from build123d import *

# Parameters (mm, degrees)
SKETCH1_R                 = 3.4
F_40_X_40L_X_R4_5_1_DEPTH = 300


with BuildPart() as part:
    # Sketch1 → 铝型材 40 X 40L X R4.5(1) (new body)
    with BuildSketch(Plane.XY.offset(-151.807228916)):
        with BuildLine():
            Line((-5.1, 20), (-5.1, 19.5))
            Line((-5.1, 19.5), (-4.1, 19.5))
            Line((-4.1, 19.5), (-4.1, 17))
            Line((-4.1, 17), (-6.1, 17))
            Line((-6.1, 17), (-6.1, 18.5))
            Line((-6.1, 18.5), (-10.3, 18.5))
            Line((-10.3, 18.5), (-10.3, 11.3))
            Line((-10.3, 11.3), (-5, 6))
            Line((-5, 6), (5, 6))
            Line((5, 6), (10.3, 11.3))
            Line((10.3, 11.3), (10.3, 18.5))
            Line((10.3, 18.5), (6.1, 18.5))
            Line((6.1, 18.5), (6.1, 17))
            Line((6.1, 17), (4.1, 17))
            Line((4.1, 17), (4.1, 19.5))
            Line((4.1, 19.5), (5.1, 19.5))
            Line((5.1, 19.5), (5.1, 20))
            Line((5.1, 20), (15.5, 20))
            ThreePointArc((15.5, 20), (18.681980515, 18.681980515), (20, 15.5))
            Line((20, 15.5), (20, 5.1))
            Line((20, 5.1), (19.5, 5.1))
            Line((19.5, 5.1), (19.5, 4.1))
            Line((19.5, 4.1), (17, 4.1))
            Line((17, 4.1), (17, 6.1))
            Line((17, 6.1), (18.5, 6.1))
            Line((18.5, 6.1), (18.5, 10.3))
            Line((18.5, 10.3), (11.3, 10.3))
            Line((11.3, 10.3), (6, 5))
            Line((6, 5), (6, -5))
            Line((6, -5), (11.3, -10.3))
            Line((11.3, -10.3), (18.5, -10.3))
            Line((18.5, -10.3), (18.5, -6.1))
            Line((18.5, -6.1), (17, -6.1))
            Line((17, -6.1), (17, -4.1))
            Line((17, -4.1), (19.5, -4.1))
            Line((19.5, -4.1), (19.5, -5.1))
            Line((19.5, -5.1), (20, -5.1))
            Line((20, -5.1), (20, -15.5))
            ThreePointArc((20, -15.5), (18.681980515, -18.681980515), (15.5, -20))
            Line((15.5, -20), (5.1, -20))
            Line((5.1, -20), (5.1, -19.5))
            Line((5.1, -19.5), (4.1, -19.5))
            Line((4.1, -19.5), (4.1, -17))
            Line((4.1, -17), (6.1, -17))
            Line((6.1, -17), (6.1, -18.5))
            Line((6.1, -18.5), (10.3, -18.5))
            Line((10.3, -18.5), (10.3, -11.3))
            Line((10.3, -11.3), (5, -6))
            Line((5, -6), (-5, -6))
            Line((-5, -6), (-10.3, -11.3))
            Line((-10.3, -11.3), (-10.3, -18.5))
            Line((-10.3, -18.5), (-6.1, -18.5))
            Line((-6.1, -18.5), (-6.1, -17))
            Line((-6.1, -17), (-4.1, -17))
            Line((-4.1, -17), (-4.1, -19.5))
            Line((-4.1, -19.5), (-5.1, -19.5))
            Line((-5.1, -19.5), (-5.1, -20))
            Line((-5.1, -20), (-15.5, -20))
            ThreePointArc((-15.5, -20), (-18.681980515, -18.681980515), (-20, -15.5))
            Line((-20, -15.5), (-20, -5.1))
            Line((-20, -5.1), (-19.5, -5.1))
            Line((-19.5, -5.1), (-19.5, -4.1))
            Line((-19.5, -4.1), (-17, -4.1))
            Line((-17, -4.1), (-17, -6.1))
            Line((-17, -6.1), (-18.5, -6.1))
            Line((-18.5, -6.1), (-18.5, -10.3))
            Line((-18.5, -10.3), (-11.3, -10.3))
            Line((-11.3, -10.3), (-6, -5))
            Line((-6, -5), (-6, 5))
            Line((-6, 5), (-11.3, 10.3))
            Line((-11.3, 10.3), (-18.5, 10.3))
            Line((-18.5, 10.3), (-18.5, 6.1))
            Line((-18.5, 6.1), (-17, 6.1))
            Line((-17, 6.1), (-17, 4.1))
            Line((-17, 4.1), (-19.5, 4.1))
            Line((-19.5, 4.1), (-19.5, 5.1))
            Line((-19.5, 5.1), (-20, 5.1))
            Line((-20, 5.1), (-20, 15.5))
            ThreePointArc((-20, 15.5), (-18.681980515, 18.681980515), (-15.5, 20))
            Line((-15.5, 20), (-5.1, 20))
        make_face()
        Circle(SKETCH1_R, mode=Mode.SUBTRACT)
        with BuildLine():
            Line((11.8, 17.5), (15, 17.5))
            ThreePointArc((15, 17.5), (16.767766953, 16.767766953), (17.5, 15))
            Line((17.5, 15), (17.5, 11.8))
            Line((17.5, 11.8), (11.8, 11.8))
            Line((11.8, 11.8), (11.8, 17.5))
        make_face(mode=Mode.SUBTRACT)
        with BuildLine():
            Line((-15, 17.5), (-11.8, 17.5))
            Line((-11.8, 17.5), (-11.8, 11.8))
            Line((-11.8, 11.8), (-17.5, 11.8))
            Line((-17.5, 11.8), (-17.5, 15))
            ThreePointArc((-17.5, 15), (-16.767766953, 16.767766953), (-15, 17.5))
        make_face(mode=Mode.SUBTRACT)
        with BuildLine():
            Line((-17.5, -11.8), (-11.8, -11.8))
            Line((-11.8, -11.8), (-11.8, -17.5))
            Line((-11.8, -17.5), (-15, -17.5))
            ThreePointArc((-15, -17.5), (-16.767766953, -16.767766953), (-17.5, -15))
            Line((-17.5, -15), (-17.5, -11.8))
        make_face(mode=Mode.SUBTRACT)
        with BuildLine():
            Line((11.8, -11.8), (17.5, -11.8))
            Line((17.5, -11.8), (17.5, -15))
            ThreePointArc((17.5, -15), (16.767766953, -16.767766953), (15, -17.5))
            Line((15, -17.5), (11.8, -17.5))
            Line((11.8, -17.5), (11.8, -11.8))
        make_face(mode=Mode.SUBTRACT)
    extrude(amount=F_40_X_40L_X_R4_5_1_DEPTH)


solid = part.part
Build history of the part. All positions in model axes, mm. A direction names the side the tool comes from. Round coordinates to 2 decimals unless told otherwise and drop trailing zeros. Write each loop counter-clockwise with the first axis right and the second up, starting at its lowest first coordinate (ties: lowest second). Pieces come first, ordered by that corner, then holes. Notation, with made-up numbers: M 83.25,45.5 L 113.25,45.5 A15 ccw 113.25,56.5 Z; hole C 21,-14 d5. An arc over 180 degrees is marked long. Answer as a JSON object with one key per item and string values. Group by question number.
(1) Cut at C-C (z = -110). Give the number of separate pieces and of enclosed holes in the cut face, and give its area (3 significant figures).
(2) Cut at A-A (x = 0). Give the cut face in (y, z).
(3) Which spindle directions (+Z, -Z, +X, -X, +Y, -Y) get a long thin tool onto all of the face, cutting with end or side? Do faces 4 (the flat face through (9, 8, -4)), 5 (the flat face through (10, -20, -4)). Say none if no direction does.
(4) Drill centre lines: L1, parallel to Y at x = 4.5, z = -18; L2, parallel to X at y = 14, z = 99; L3, parallel to Y at x = -15.5, z = 5.5. Where is each one in solid material? Low to high.
(5) Mould opens along Y. For faces 1 (the flat face through (-11.8, -15, -4)), 2 (the flat face through (-3, 3, -151.807)), 3 (the flat face through (-10, -20, -4)) say: pulls with the +Y half, pulls with the -Y half, needs draft (parallel to the pull), parting line crosses it, or undercut.
(6) Flat gauge pins, fed straight in: pin 1 (1 mm diameter, centred on y = -0.5, z = -24.5, fed in from -X); pin 2 (0.5 mm diameter, centred on y = -4.5, z = 9.5, fed in from +X). Where does each tip first touch, or does it go through?
Responses:
{
 "1": {"separate pieces": "1", "enclosed holes": "5", "area": "475 mm2"},
 "2": {"outline": "M -6,-151.81 L -3.4,-151.81 L -3.4,148.19 L -6,148.19 Z; M 3.4,-151.81 L 6,-151.81 L 6,148.19 L 3.4,148.19 Z"},
 "3": {"face 4": "+Z, -Z", "face 5": "+Z, -Z, +X, -X, -Y"},
 "4": {"L1": "y = -19.5 to -17, -6 to 6, 17 to 19.5", "L2": "x = -20 to -17.5, -11.8 to -10.3, 10.3 to 11.8, 17.5 to 20", "L3": "y = -20 to -17.45, -11.8 to -10.3, 10.3 to 11.8, 17.45 to 20"},
 "5": {"face 1": "undercut", "face 2": "needs draft", "face 3": "pulls with the -Y half"},
 "6": {"pin 1": "stops at x = -6", "pin 2": "stops at x = 19.5"}
}
